The listing builds one solid part. Answer for the finished solid, in the listing's coordinates (mm). A direction names the side the tool comes from. Give positions to 0.01 mm unless a question says otherwise; leave off trailing zeros. Write each loop counter-clockwise with the first axis right and the second up, starting at its lowest first coordinate (ties: lowest second). Pieces come first, ordered by that corner, then holes. Notation, with made-up numbers: (29, 23) -> (39, 23) arc R31 ccw to (39, 48) -> close; hole circle Ø10 at (40, 31.5). An arc over 180 degrees is marked (long way). Write each question's results on one line, items separated by ' | '. Start each with the question number.
from build123d import *

# Parameters (mm, degrees)
F0_R     = 3.5
F1_DEPTH = 340


with BuildPart() as f1:
    # F0 (on Top) → F1 (new body)
    with BuildSketch(Plane.XY):
        Polygon((-4, 15), (-15, 15), (-15, 4), (-12, 4), (-12, 10), (-6, 4), (-6, 0), (-6, -4), (-12, -10), (-12, -4), (-15, -4), (-15, -15), (-4, -15), (-4, -12), (-10, -12), (-4, -6), (0, -6), (4, -6), (10, -12), (4, -12), (4, -15), (15, -15), (15, -4), (12, -4), (12, -10), (6, -4), (6, 0), (6, 4), (12, 10), (12, 4), (15, 4), (15, 15), (4, 15), (4, 12), (10, 12), (4, 6), (0, 6), (-4, 6), (-10, 12), (-4, 12), align=None)
        Circle(F0_R, mode=Mode.SUBTRACT)
    extrude(amount=F1_DEPTH)


solid = f1.part
1. Each of these flat-tipped pins is pushed along its axis until it touches: pin 1 Ø2 at (x, y) = (10, 5) entering from +Z; pin 2 Ø4 at (x, y) = (-3.5, -1) entering from -Z; pin 3 Ø1.5 at (y, z) = (-3, 132.5) entering from -X; pin 4 Ø2.5 at (x, z) = (0.5, 163.5) entering from -Y. Where does it stop, or does it pass through?
2. A tool of negligible diameter and unlimited length cuts with its end or side. For faces 1 (the flat face through (15, 9, 168)), 2 (the flat face through (0, 6, 168)), 3 (the flat face through (-6, 0, 168)), from which of +Z, -Z, +X, -X, +Y, -Y can it reach the whole face along a straight path? Write none if from no direction.
3. Section A-A (y = 0) is taken. Write down the section's boundary in (x, z), then the cut area to 3 significant figures.
4. The mould has two halves that part along Y. Classify faces 4 (the flat face through (-10, -15, 168)), 5 (the flat face through (12, -7, 168)), 6 (the flat face through (0, 4, 340)): pulls with the +Y half, pulls with the -Y half, needs draft (parallel to the pull), parting line crosses it, or undercut.
5. Consider probe 1 along Y at (x, z) = (0, 236.5); probe 2 along X at (y, z) = (-8, 241); probe 3 along X at (y, z) = (0.5, 319). Determine where each line is inside the solid, lowest interval first. Write a range as [from, to].
Results:
1) pin 1: passes through | pin 2: stops at z = 0 | pin 3: stops at x = -6 | pin 4: stops at y = -6
2) face 1: +Z, -Z, +X, +Y, -Y | face 2: +Z, -Z, +Y | face 3: +Z, -Z, -X
3) outline: (-6, 0) -> (-3.5, 0) -> (-3.5, 340) -> (-6, 340) -> close; (3.5, 0) -> (6, 0) -> (6, 340) -> (3.5, 340) -> close | area: 1,700 mm²
4) face 4: pulls with the -Y half | face 5: undercut | face 6: needs draft
5) probe 1: y = [-6, -3.5], [3.5, 6] | probe 2: x = [-15, -12], [-10, -6], [6, 10], [12, 15] | probe 3: x = [-6, -3.46], [3.46, 6]
